The listing builds one solid part. Answer for the finished solid, in the listing's coordinates (mm). Face numbers are marked on the shaded views. A direction names the side the tool comes from. Round coordinates to 2 decimals unless told otherwise and drop trailing zeros. Order: outer loops, then holes, each group sorted by start corner. A loop starts at its lowest first (then second) coordinate and runs counter-clockwise, first axis right, second up. Notation, with made-up numbers: M 11.25,-12 L 66.25,-12 A22 cw 66.25,22 Z; hole C 53,-1 d11. An arc over 180 degrees is marked long. Put each result on its own line as item: value. Start each with the question number.
1. The part is cut by section B-B (x = 19.5). Give the vertices of the cut face in (y, z) (3 decimals).
2. Which of the six approach directions +Z, -Z, +X, -X, +Y, -Y give full straight-line access (tool end or side, diameter ignored) to the marked faces 4, 5 and 6?
3. The part is cut by section D-D (x = 0.5). Give the vertices of the cut face in (y, z) (3 decimals).
4. Each of these flat-tipped pins is pushed along its axis until it touches: pin 1 Ø4 at (x, y) = (4, -26) entering from +Z (3 decimals); pin 2 Ø12.5 at (x, y) = (1, -16) entering from -Z (3 decimals); pin 3 Ø10.5 at (x, y) = (0, -31) entering from +Z (3 decimals). Where does it stop, or does it pass through?
5. Consider line 1 (Y direction, x = 24.5, z = -15); line 2 (Y direction, x = -5, z = 4.5) (3 decimals); line 3 (Z direction, x = -2, y = -33) (3 decimals). Determine where each line is inside the solid, lowest interval first.
6. The mould has two halves that part along X. Classify the marked faces 1, 2 and 3: +X half, -X half, draft (parallel to the pull), parting line (faces both ways), or undercut.
7. The part is cut by section C-C (y = -31). Give the vertices of the cut face in (x, z) (3 decimals).
8. The part is cut by section A-A (z = 5.5). Give the vertices of the cut face in (x, y) (3 decimals).
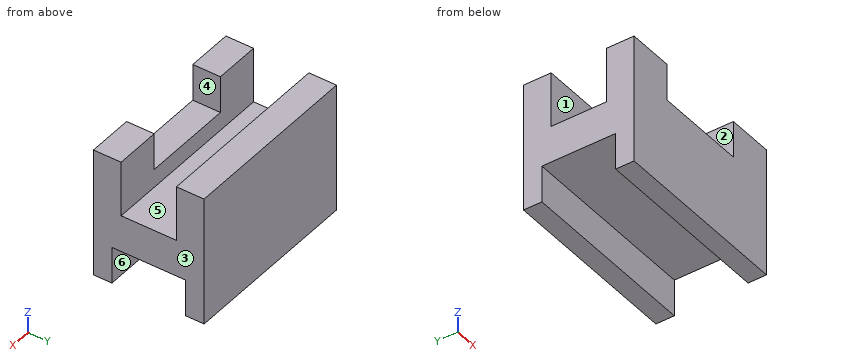
from build123d import *

# Parameters (mm, degrees)
F0_W     = 63.5
F0_H     = 44.45
F1_DEPTH = 38.1
F2_W     = 63.5
F2_H     = 19.05
F3_DEPTH = 19.05
F4_W     = 63.5
F4_H     = 25.4
F5_DEPTH = 12.7
F6_W     = 31.75
F6_H     = 9.525
F7_DEPTH = 12.7


with BuildPart() as f1:
    # F0 (on Front) → F1 (new body)
    with BuildSketch(Plane.XZ):
        Rectangle(F0_W, F0_H)
    extrude(amount=F1_DEPTH)

    # F2 (on face) → F3 (cut)
    with BuildSketch(Plane.XY.offset(22.225)):
        with Locations((0, -19.05)):
            Rectangle(F2_W, F2_H)
    extrude(amount=-F3_DEPTH, mode=Mode.SUBTRACT)

    # F4 (on face) → F5 (cut)
    with BuildSketch(Plane(origin=(0, 0, -22.225), x_dir=(1, 0, 0), z_dir=(0, 0, -1))):
        with Locations((0, 19.05)):
            Rectangle(F4_W, F4_H)
    extrude(amount=-F5_DEPTH, mode=Mode.SUBTRACT)

    # F6 (on face) → F7 (cut)
    with BuildSketch(Plane.XY.offset(22.225)):
        with Locations((0, -33.3375)):
            Rectangle(F6_W, F6_H)
    extrude(amount=-F7_DEPTH, mode=Mode.SUBTRACT)


solid = f1.part
Resolved:
1. outline: M -38.1,-22.225 L -31.75,-22.225 L -31.75,-9.525 L -6.35,-9.525 L -6.35,-22.225 L 0,-22.225 L 0,22.225 L -9.525,22.225 L -9.525,3.175 L -28.575,3.175 L -28.575,22.225 L -38.1,22.225 Z
2. face 4: +Z, -Y
2. face 5: +Z, +X, -X
2. face 6: -Z, +X, -X
3. outline: M -38.1,-22.225 L -31.75,-22.225 L -31.75,-9.525 L -6.35,-9.525 L -6.35,-22.225 L 0,-22.225 L 0,22.225 L -9.525,22.225 L -9.525,3.175 L -28.575,3.175 L -28.575,9.525 L -38.1,9.525 Z
4. pin 1: z = 3.175
4. pin 2: z = -9.525
4. pin 3: z = 9.525
5. line 1: -38.1 to -31.75, -6.35 to 0
5. line 2: -38.1 to -28.575, -9.525 to 0
5. line 3: -22.225 to 9.525
6. face 1: draft
6. face 2: undercut
6. face 3: +X half
7. outline: M -31.75,-9.525 L 31.75,-9.525 L 31.75,22.225 L 15.875,22.225 L 15.875,9.525 L -15.875,9.525 L -15.875,22.225 L -31.75,22.225 Z
8. outline: M -31.75,-38.1 L 31.75,-38.1 L 31.75,-28.575 L -31.75,-28.575 Z; M -31.75,-9.525 L 31.75,-9.525 L 31.75,0 L -31.75,0 Z
